```python
from build123d import *

# Parameters (mm, degrees)
SKETCH_1_R          = 15.8
EXTRUDE_1_DEPTH     = 4.4
CUT_EXTRUDE_2_DEPTH = 4.4
SKETCH_4_R          = 19.4
SKETCH_4_R_2        = 15.8
EXTRUDE_2_DEPTH     = 4.4
EXTRUDE_3_DEPTH     = 4.4
SKETCH_6_W          = 15
SKETCH_6_H          = 38.8
CUT_EXTRUDE_3_DEPTH = 2.2


with BuildPart() as part:
    # 草圖1 → 填料-伸長1 (new body)
    with BuildSketch(Plane(origin=(0, 0, 0), x_dir=(1, 0, 0), z_dir=(0, 1, 0))):
        Circle(SKETCH_1_R)
    extrude(amount=EXTRUDE_1_DEPTH)

    # 草圖3 → 除料-伸長2 (cut)
    with BuildSketch(Plane.XZ):
        with BuildLine():
            Line((-1.5, 14.3), (-3.4, 7.272575881))
            Line((-3.4, 7.272575881), (-3.650072203, 6.322110506))
            Line((-3.650072203, 6.322110506), (-4.598235464, 6.580774314))
            Line((-4.598235464, 6.580774314), (-11.634163274, 8.449038106))
            ThreePointArc((-11.634163274, 8.449038106), (-12.772391842, 8.598888739), (-13.68320138, 7.9))
            ThreePointArc((-13.68320138, 7.9), (-13.833052014, 6.761771432), (-13.134163274, 5.850961894))
            Line((-13.134163274, 5.850961894), (-7.998235464, 0.691801568))
            Line((-7.998235464, 0.691801568), (-7.300144405, 0))
            Line((-7.300144405, 0), (-7.998235464, -0.691801568))
            Line((-7.998235464, -0.691801568), (-13.134163274, -5.850961894))
            ThreePointArc((-13.134163274, -5.850961894), (-13.833052014, -6.761771432), (-13.68320138, -7.9))
            ThreePointArc((-13.68320138, -7.9), (-12.772391842, -8.598888739), (-11.634163274, -8.449038106))
            Line((-11.634163274, -8.449038106), (-4.598235464, -6.580774314))
            Line((-4.598235464, -6.580774314), (-3.650072203, -6.322110506))
            Line((-3.650072203, -6.322110506), (-3.4, -7.272575881))
            Line((-3.4, -7.272575881), (-1.5, -14.3))
            ThreePointArc((-1.5, -14.3), (-1.060660172, -15.360660172), (0, -15.8))
            ThreePointArc((0, -15.8), (1.060660172, -15.360660172), (1.5, -14.3))
            Line((1.5, -14.3), (3.4, -7.272575881))
            Line((3.4, -7.272575881), (3.650072203, -6.322110506))
            Line((3.650072203, -6.322110506), (4.598235464, -6.580774314))
            Line((4.598235464, -6.580774314), (11.634163274, -8.449038106))
            ThreePointArc((11.634163274, -8.449038106), (12.772391842, -8.598888739), (13.68320138, -7.9))
            ThreePointArc((13.68320138, -7.9), (13.833052014, -6.761771432), (13.134163274, -5.850961894))
            Line((13.134163274, -5.850961894), (7.998235464, -0.691801568))
            Line((7.998235464, -0.691801568), (7.300144405, 0))
            Line((7.300144405, 0), (7.998235464, 0.691801568))
            Line((7.998235464, 0.691801568), (13.134163274, 5.850961894))
            ThreePointArc((13.134163274, 5.850961894), (13.833052014, 6.761771432), (13.68320138, 7.9))
            ThreePointArc((13.68320138, 7.9), (12.772391842, 8.598888739), (11.634163274, 8.449038106))
            Line((11.634163274, 8.449038106), (4.598235464, 6.580774314))
            Line((4.598235464, 6.580774314), (3.650072203, 6.322110506))
            Line((3.650072203, 6.322110506), (3.4, 7.272575881))
            Line((3.4, 7.272575881), (1.5, 14.3))
            ThreePointArc((1.5, 14.3), (1.060660172, 15.360660172), (0, 15.8))
            ThreePointArc((0, 15.8), (-1.060660172, 15.360660172), (-1.5, 14.3))
        make_face()
    extrude(amount=-CUT_EXTRUDE_2_DEPTH, mode=Mode.SUBTRACT)

    # 草圖4 → 填料-伸長2 (add)
    with BuildSketch(Plane(origin=(0, 0, 0), x_dir=(1, 0, 0), z_dir=(0, 1, 0))):
        Circle(SKETCH_4_R)
        Circle(SKETCH_4_R_2, mode=Mode.SUBTRACT)
    extrude(amount=EXTRUDE_2_DEPTH)

    # 草圖5 → 填料-伸長3 (add)
    with BuildSketch(Plane(origin=(0, 4.4, 0), x_dir=(1, 0, 0), z_dir=(0, 1, 0))):
        with BuildLine():
            Line((0, 19.4), (-160, 19.4))
            Line((-160, 19.4), (-160, -19.4))
            Line((-160, -19.4), (0, -19.4))
            ThreePointArc((0, -19.4), (-19.4, 0), (0, 19.4))
        make_face()
    extrude(amount=-EXTRUDE_3_DEPTH)

    # 草圖6 → 除料-伸長3 (cut)
    with BuildSketch(Plane(origin=(0, 4.4, 0), x_dir=(1, 0, 0), z_dir=(0, 1, 0))):
        with Locations((-152.5, 0)):
            Rectangle(SKETCH_6_W, SKETCH_6_H)
    extrude(amount=-CUT_EXTRUDE_3_DEPTH, mode=Mode.SUBTRACT)


solid = part.part
```
Can you work these out from the model? Positions are in its coordinate system, mm. A direction names the side the tool comes from. Coordinates: 2 decimals unless noted, no trailing zeros. Loops run counter-clockwise (first coordinate to the right, second up) from the corner with the lowest first, then second, coordinate; pieces in that order, holes last.
1) I need wall thicknesses on probe 1 along Z at (x, y) = (-9.5, 1.2); probe 2 along Z at (x, y) = (-13.5, 4.15); probe 3 along X at (y, z) = (0.6, -6). Which ranges of each line are inside material? Lowest first, please.
2) Which directions (+Z, -Z, +X, -X, +Y, -Y) give clear straight access to the entire face, cutting with the end or side of a thin tool? Please do faces 4 (the flat face through (-153, 2.2, 0)), 5 (the flat face through (-79, 2, -19.4)), 6 (the flat face through (-8.067, 2.169, 7.502)).
3) Thinking about a two-plate mould opening in X: for faces 1 (the flat face through (-72, 0, 0)), 2 (the cylindrical face through (19.395, 2.169, 0.427)), 3 (the flat face through (10.602, 2.169, -3.307)), which applies, pulls with the +X half, pulls with the -X half, needs draft (parallel to the pull), parting line crosses it, or undercut?
4) Imagine slicing it at A-A on z = 2.5. List the corners of the cut face in (x, y) for me, plus the area to 3 significant figures.
5) For pin 1 (7.5 mm diameter, centred on x = -152, z = -5.5, fed in from +Y); pin 2 (0.7 mm diameter, centred on y = 4, z = -8.5, fed in from -X), each with a flat end and sliding along its axis, tell me the tip position at first contact or that it passes through.
Completed:
1. probe 1: z = -19.4 to -7.88, -2.2 to 2.2, 7.88 to 19.4
1. probe 2: z = -19.4 to -8.15, -6.15 to 6.15, 8.15 to 19.4
1. probe 3: x = -160 to -13.35, 13.35 to 18.45
2. face 4: +Z, -Z, -X, +Y
2. face 5: -Z, +X, -X, +Y, -Y
2. face 6: +Y, -Y
3. face 1: needs draft
3. face 2: pulls with the +X half
3. face 3: undercut
4. outline: (-160, 0) - (-9.8, 0) - (-9.8, 4.4) - (-145, 4.4) - (-145, 2.2) - (-160, 2.2) - close; (9.8, 0) - (19.24, 0) - (19.24, 4.4) - (9.8, 4.4) - close
4. area: 669 mm2
5. pin 1: stops at y = 2.2
5. pin 2: stops at x = -145
